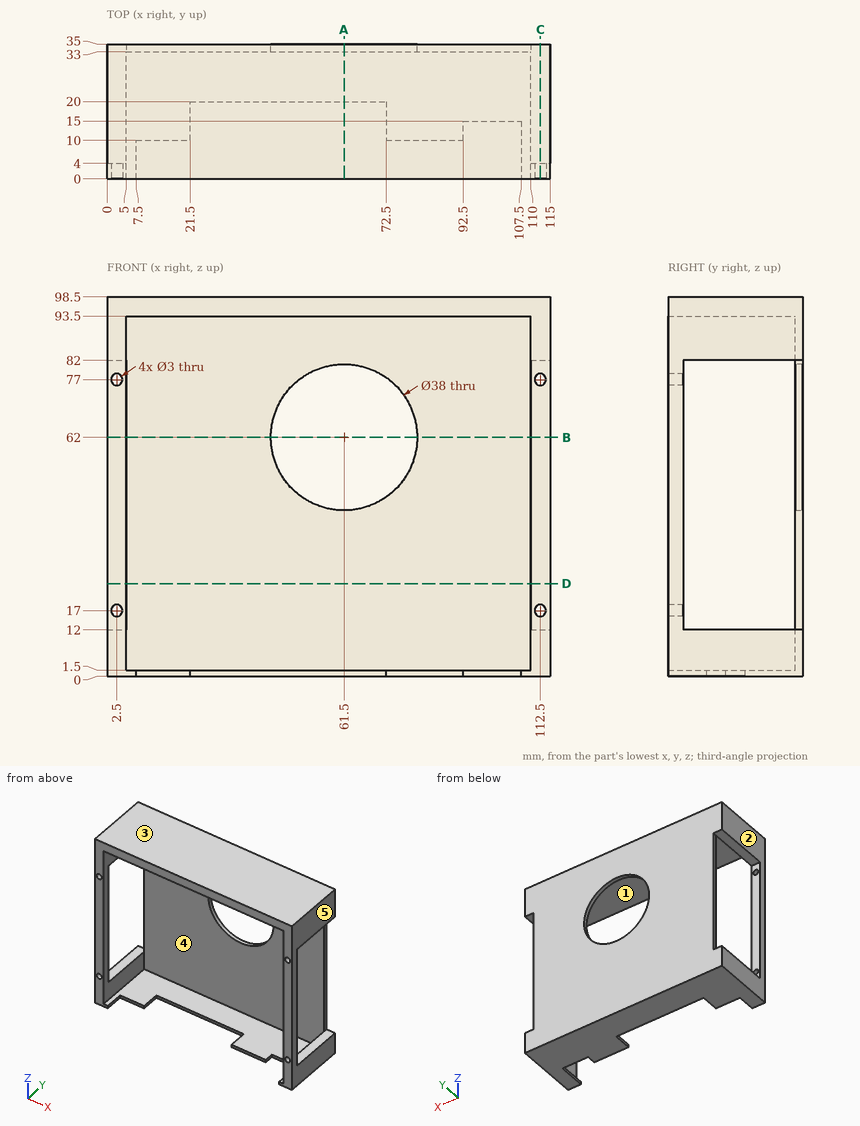
For this review, use the dimensioned drawing (mm, ordinates from the lowest corner) and the shaded views. A direction names the side the tool comes from. Round coordinates to 2 decimals unless told otherwise and drop trailing zeros. Write each loop counter-clockwise with the first axis right and the second up, starting at its lowest first coordinate (ties: lowest second). Pieces come first, ordered by that corner, then holes. Notation, with made-up numbers: (64.25, 46) - (80.25, 46) arc R13 cw to (80.25, 54) - close; hole circle Ø3 at (87.25, 87.25). An arc over 180 degrees is marked (long way). One line per item, written item: value. Start each with the question number.
1. Consider section B-B on z = 62. Write out the cut boundary in (x, y).
2. Consider section C-C on x = 112.5. Write out the cut boundary in (y, z).
3. Consider section A-A on x = 61.5. Write out the cut boundary in (y, z).
4. Machinability: for the marked faces 1 and 2, which of the approach directions +Z, -Z, +X, -X, +Y, -Y give a long, thin tool a straight path to every point of the face, cutting with its end or side? Answer none if there is none.
5. Clearance check with flat-ended pins moving along their axes: P1, Ø0.8, axis at x = 85, z = 0.5, coming from the -Y side; P2, Ø2.5, axis at x = 1.5, z = 59, coming from the +Y side; P3, Ø1.2, axis at y = 12.5, z = 0.5, coming from the -X side; P4, Ø1.2, axis at x = 97, z = 1, coming from the -Y side. State where each tip first meets the part, or that it passes through.
6. Consider section D-D on z = 24. Write out the cut boundary in (x, y), and give its area (3 significant figures).
7. The part is to be moulded in two halves that separate along X. For the marked faces 3, 4 and 5, say which applies: released by +X, released by -X, zero draft, split by the parting line, or undercut.
8. To check wall thickness, follow L1, parallel to X at y = 2, z = 77; L2, parallel to Z at x = 112.5, y = 1.9; L3, parallel to Z at x = 93, y = 22.5. State the ranges of each line that lie inside material, in increasing order. Write a range as from..to.
Checks:
1. outline: (0, 0) - (5, 0) - (5, 4) - (0, 4) - close; (5, 33) - (42.5, 33) - (42.5, 35) - (5, 35) - close; (80.5, 33) - (110, 33) - (110, 35) - (80.5, 35) - close; (110, 0) - (115, 0) - (115, 4) - (110, 4) - close
2. outline: (0, 0) - (35, 0) - (35, 12) - (4, 12) - (4, 15.5) - (0, 15.5) - close; (0, 18.5) - (4, 18.5) - (4, 75.5) - (0, 75.5) - close; (0, 78.5) - (4, 78.5) - (4, 82) - (35, 82) - (35, 98.5) - (0, 98.5) - close
3. outline: (0, 93.5) - (33, 93.5) - (33, 81) - (35, 81) - (35, 98.5) - (0, 98.5) - close; (20, 0) - (35, 0) - (35, 43) - (33, 43) - (33, 1.5) - (20, 1.5) - close
4. face 1: -Y
4. face 2: +Z, -Z, -X, +Y, -Y
5. P1: stops at y = 10
5. P2: stops at y = 4
5. P3: stops at x = 0
5. P4: stops at y = 15
6. outline: (0, 0) - (5, 0) - (5, 4) - (0, 4) - close; (5, 33) - (110, 33) - (110, 35) - (5, 35) - close; (110, 0) - (115, 0) - (115, 4) - (110, 4) - close
6. area: 250 mm^2
7. face 3: zero draft
7. face 4: undercut
7. face 5: released by +X
8. L1: x = 0..1, 4..5, 110..111, 114..115
8. L2: z = 0..15.5, 18.5..75.5, 78.5..98.5
8. L3: z = 0..1.5, 93.5..98.5
